For this review, take the finished solid that the model builds, in its own axes (mm). A direction names the side the tool comes from. Round coordinates to 2 decimals unless told otherwise and drop trailing zeros. Order: outer loops, then holes, each group sorted by start corner. A loop starts at its lowest first (then second) coordinate and runs counter-clockwise, first axis right, second up. Notation, with made-up numbers: (64, 63) -> (95, 63) arc R29 ccw to (95, 102) -> close; hole circle Ø4 at (86, 67.5). An arc over 180 degrees is marked (long way). Answer in a Markdown table with one row per item.
```python
from build123d import *

# Parameters (mm, degrees)
SKETCH1_R           = 8.375
SKETCH1_R_2         = 5.375
BOSS_EXTRUDE1_DEPTH = 100
BOSS_EXTRUDE2_DEPTH = 75


with BuildPart() as part:
    # Sketch1 → Boss-Extrude1 (new body)
    with BuildSketch(Plane(origin=(0, 0, 0), x_dir=(1, 0, 0), z_dir=(0, 1, 0))):
        Circle(SKETCH1_R)
        Circle(SKETCH1_R_2, mode=Mode.SUBTRACT)
    extrude(amount=BOSS_EXTRUDE1_DEPTH)

    # Sketch2 → Boss-Extrude2 (add)
    with BuildSketch(Plane(origin=(0, 0, 0), x_dir=(1, 0, 0), z_dir=(0, 1, 0))):
        with BuildLine():
            Line((8.445467678, 1.5), (8.239576749, 1.5))
            ThreePointArc((8.239576749, 1.5), (8.375, 0), (8.239576749, -1.5))
            Line((8.239576749, -1.5), (8.445467678, -1.5))
            ThreePointArc((8.445467678, -1.5), (10.909272228, -8.64142208), (16.375, -13.856406461))
            Line((16.375, -13.856406461), (17.875, -11.258330249))
            ThreePointArc((17.875, -11.258330249), (11.375, 0), (17.875, 11.258330249))
            Line((17.875, 11.258330249), (16.375, 13.856406461))
            ThreePointArc((16.375, 13.856406461), (10.909272228, 8.64142208), (8.445467678, 1.5))
        make_face()
    extrude(amount=BOSS_EXTRUDE2_DEPTH)


solid = part.part
```
Q1. Take a section at D-D, the plane z = 4.5. Write out the cut boundary in (x, y).
Answer key:
| item | result |
|---|---|
| outline | (-7.06, 0) -> (-2.94, 0) -> (-2.94, 100) -> (-7.06, 100) -> close; (2.94, 0) -> (7.06, 0) -> (7.06, 100) -> (2.94, 100) -> close; (9.02, 0) -> (12.18, 0) -> (12.18, 75) -> (9.02, 75) -> close |
Q2. To check wall thickness, follow probe 1 along Z at (x, y) = (0, 45) (3 decimals); probe 2 along X at (y, z) = (70, 0) (3 decimals). State the ranges of each line that lie inside material, in increasing order.
Answer key:
| item | result |
|---|---|
| probe 1 | z = -8.375 to -5.375, 5.375 to 8.375 |
| probe 2 | x = -8.375 to -5.375, 5.375 to 11.375 |
Q3. Clearance check with flat-ended pins moving along their axes: pin 1 Ø5 at (x, y) = (2.5, 51.5) entering from +Z (3 decimals); pin 2 Ø12 at (y, z) = (62, -7.5) entering from -X; pin 3 Ø5 at (x, y) = (-5.5, 73) entering from -Z; pin 4 Ø2 at (x, z) = (2, -2.5) entering from -Y. State where each tip first meets the part, or that it passes through.
Answer key:
| item | result |
|---|---|
| pin 1 | stops at z = 8.375 |
| pin 2 | stops at x = -8.24 |
| pin 3 | stops at z = -7.82 |
| pin 4 | passes through |
Q4. Take a section at C-C, the plane x = 0. Write out the cut boundary in (y, z) (3 decimals), then the cut area to 3 significant figures.
Answer key:
| item | result |
|---|---|
| outline | (0, -8.375) -> (100, -8.375) -> (100, -5.375) -> (0, -5.375) -> close; (0, 5.375) -> (100, 5.375) -> (100, 8.375) -> (0, 8.375) -> close |
| area | 600 mm^2 |
Q5. Take a section at B-B, the plane z = 0. Write out the cut boundary in (x, y) (3 decimals).
Answer key:
| item | result |
|---|---|
| outline | (-8.375, 0) -> (-5.375, 0) -> (-5.375, 100) -> (-8.375, 100) -> close; (5.375, 0) -> (11.375, 0) -> (11.375, 75) -> (8.375, 75) -> (8.375, 100) -> (5.375, 100) -> close |
Q6. Take a section at A-A, the plane y = 43. Write out the cut boundary in (x, z) (3 decimals), then the cut area to 3 significant figures.
Answer key:
| item | result |
|---|---|
| outline | (8.24, -1.5) -> (8.445, -1.5) arc R16 ccw to (16.375, -13.856) -> (17.875, -11.258) arc R13 cw to (17.875, 11.258) -> (16.375, 13.856) arc R16 ccw to (8.445, 1.5) -> (8.24, 1.5) arc R8.375 ccw (long way) to start; hole circle Ø10.75 at (0, 0) |
| area | 221 mm^2 |
Q7. Tool access review of faces 4 (the face through (10.967, 36.975, -8.731)), 5 (the face through (1.7, 100, 5.5)), 6 (the face through (10.85, 36.98, 8.55)): name each direction out of +Z, -Z, +X, -X, +Y, -Y from which nothing blocks a thin tool from reaching the whole face with its end or side.
Answer key:
| item | result |
|---|---|
| face 4 | -Z, +Y, -Y |
| face 5 | +Z, -Z, +X, -X, +Y |
| face 6 | +Z, +Y, -Y |
Q8. The part is to be moulded in two halves that separate along X. For faces 1 (the face through (17.1, 37, 12.6)), 2 (the face through (6, 0, -1)), 3 (the face through (7.988, 49.3, -2.516)), say which applies: +X half, -X half, draft (parallel to the pull), parting line (faces both ways), or undercut.
Answer key:
| item | result |
|---|---|
| face 1 | +X half |
| face 2 | draft |
| face 3 | undercut |
